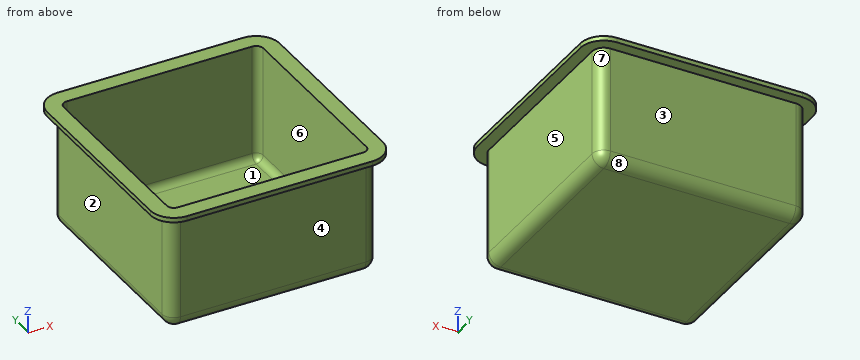
Autodesk Inventor part; units mm, degrees
ref_plane "YZ Plane" through (0, 0, 0) normal (1, 0, 0) x (0, 1, 0)
ref_plane "XZ Plane" through (0, 0, 0) normal (0, 1, 0) x (-1, 0, 0)
ref_plane "XY Plane" through (0, 0, 0) normal (0, 0, 1) x (1, 0, 0)
sketch "Sketch1" plane through (0, 0, 0) normal (0, 0, 1) x (1, 0, 0)
  line L0 (-39.5, -44.5) -> (39.5, -44.5)
  line L1 (44.5, -39.5) -> (44.5, 39.5)
  line L2 (39.5, 44.5) -> (-39.5, 44.5)
  line L3 (-44.5, 39.5) -> (-44.5, -39.5)
  line L4 (-44.5, -44.5) -> (44.5, 44.5) construction
  line L5 (44.5, -44.5) -> (-44.5, 44.5) construction
  arc A0 (-39.5, 44.5) -> (-44.5, 39.5) centre (-39.5, 39.5) ccw
  arc A1 (44.5, 39.5) -> (39.5, 44.5) centre (39.5, 39.5) ccw
  arc A2 (39.5, -44.5) -> (44.5, -39.5) centre (39.5, -39.5) ccw
  arc A3 (-44.5, -39.5) -> (-39.5, -44.5) centre (-39.5, -39.5) ccw
  line L6 (-39.5, 42.5) -> (39.5, 42.5)
  arc A4 (42.5, 39.5) -> (39.5, 42.5) centre (39.5, 39.5) ccw
  line L7 (42.5, 39.5) -> (42.5, -39.5)
  arc A5 (39.5, -42.5) -> (42.5, -39.5) centre (39.5, -39.5) ccw
  line L8 (39.5, -42.5) -> (-39.5, -42.5)
  arc A6 (-42.5, -39.5) -> (-39.5, -42.5) centre (-39.5, -39.5) ccw
  line L9 (-42.5, -39.5) -> (-42.5, 39.5)
  arc A7 (-39.5, 42.5) -> (-42.5, 39.5) centre (-39.5, 39.5) ccw
  line L10 (-49.5, -39.5) -> (-49.5, 39.5)
  arc A8 (-39.5, 49.5) -> (-49.5, 39.5) centre (-39.5, 39.5) ccw
  line L11 (-39.5, 49.5) -> (39.5, 49.5)
  arc A9 (49.5, 39.5) -> (39.5, 49.5) centre (39.5, 39.5) ccw
  line L12 (49.5, 39.5) -> (49.5, -39.5)
  arc A10 (39.5, -49.5) -> (49.5, -39.5) centre (39.5, -39.5) ccw
  line L13 (39.5, -49.5) -> (-39.5, -49.5)
  arc A11 (-49.5, -39.5) -> (-39.5, -49.5) centre (-39.5, -39.5) ccw
  point P0 (0, 0)
  dimension "d0" = 89
  dimension "d1" = 89
  dimension "d2" = 5
  dimension "d3" = 2
  dimension "d4" = 5
extrude "Extrusion1" add sketch "Sketch1" against normal blind 52 contours A3 L3 A0 L2 A1 L1 A2 L0 | L6 A4 L7 A5 L8 A6 L9 A7
extrude "Extrusion2" cut sketch "Sketch1" against normal blind 50 contours L6 A4 L7 A5 L8 A6 L9 A7
extrude "Extrusion3" add sketch "Sketch1" against normal blind 2 contours L10 A8 L11 A9 L12 A10 L13 A11
fillet "Fillet1" radius 5 8 edges at (43.0355, 43.0355, -52) (44.5, 0, -52) (43.0355, -43.0355, -52) (0, -44.5, -52) (-43.0355, -43.0355, -52) (-44.5, 0, -52) (-43.0355, 43.0355, -52) (0, 44.5, -52)
fillet "Fillet2" radius 3 8 edges at (-41.6213, -41.6213, -50) (-42.5, 0, -50) (-41.6213, 41.6213, -50) (0, 42.5, -50) (41.6213, 41.6213, -50) (42.5, 0, -50) (41.6213, -41.6213, -50) (0, -42.5, -50)
properties part number "base" material "ABS Plastic"
CAD build for the part. Positions are in the model's coordinates, mm. Face numbers are marked on the shaded views. A direction names the side the tool comes from. Coordinates: 2 decimals unless noted, no trailing zeros. Write each loop counter-clockwise with the first axis right and the second up, starting at its lowest first coordinate (ties: lowest second). Pieces come first, ordered by that corner, then holes. Notation, with made-up numbers: M 71.5,77 L 89.5,77 A26 cw 89.5,110 Z; hole C -27,63 d8. An arc over 180 degrees is marked long. Return JSON: item names as keys, results as strings.
Item 1: Which spindle directions (+Z, -Z, +X, -X, +Y, -Y) get a long thin tool onto all of the face, cutting with end or side? Do the marked faces 1, 2, 3, 4 and 5. Say none if no direction does.
Findings below:
{"face 1": "+Z", "face 2": "-Z, -X, +Y, -Y", "face 3": "-Z, +X, -X, +Y", "face 4": "-Z, +X, -X, -Y", "face 5": "-Z, +X, +Y, -Y"}
Item 2: Drop flat-ended pins along their axis: pin 1 Ø3 at (x, z) = (-26.5, -42.5) entering from +Y; pin 2 Ø13.5 at (y, z) = (16.5, -28.5) entering from -X; pin 3 Ø3 at (x, y) = (26, -37) entering from +Z. Give the stop position or say it passes through.
Findings below:
{"pin 1": "stops at y = 44.5", "pin 2": "stops at x = -44.5", "pin 3": "stops at z = -50"}
Item 3: Slice it at B-B, the plane x = -35. Write the cut outline in (y, z).
Findings below:
{"outline": "M -49.5,-2 L -44.5,-2 L -44.5,-47 A5 ccw -39.5,-52 L 39.5,-52 A5 ccw 44.5,-47 L 44.5,-2 L 49.5,-2 L 49.5,0 L 42.5,0 L 42.5,-47 A3 cw 39.5,-50 L -39.5,-50 A3 cw -42.5,-47 L -42.5,0 L -49.5,0 Z"}
Item 4: Slice it at A-A, the plane z = -44. Write the cut outline in (x, y), and give its area (3 significant figures).
Findings below:
{"outline": "M -44.5,-39.5 A5 ccw -39.5,-44.5 L 39.5,-44.5 A5 ccw 44.5,-39.5 L 44.5,39.5 A5 ccw 39.5,44.5 L -39.5,44.5 A5 ccw -44.5,39.5 Z; hole M -42.5,-39.5 A3 ccw -39.5,-42.5 L 39.5,-42.5 A3 ccw 42.5,-39.5 L 42.5,39.5 A3 ccw 39.5,42.5 L -39.5,42.5 A3 ccw -42.5,39.5 Z", "area": "682 mm2"}
Item 5: Probe line 1 (Y direction, x = 36, z = -19); line 2 (Z direction, x = -35, y = -22.5). List the from-to ranges inside material, lowest first. Write a range as from..to.
Findings below:
{"line 1": "y = -44.5..-42.5, 42.5..44.5", "line 2": "z = -52..-50"}
Item 6: Two-plate mould, pull along X, no slides. Class the marked faces 6, 7 and 8: +X half, -X half, draft (parallel to the pull), parting line (faces both ways), or undercut.
Findings below:
{"face 6": "undercut", "face 7": "+X half", "face 8": "draft"}
